For this review, take the finished solid that the model builds, in its own axes (mm). A direction names the side the tool comes from. Coordinates: 2 decimals unless noted, no trailing zeros. Write each loop counter-clockwise with the first axis right and the second up, starting at its lowest first coordinate (ties: lowest second). Pieces come first, ordered by that corner, then holes. Notation, with made-up numbers: (43, -28) -> (82, -28) arc R5 cw to (82, -24) -> close; hole circle Ø4 at (40.25, 27). An arc over 180 degrees is marked (long way). One line per item, written item: value. Start each with the question number.
1) For probe 1 along Y at (x, z) = (-44.5, 2.75); probe 2 along Y at (x, z) = (-35.5, 1); probe 3 along X at (y, z) = (11.5, 0.6), list the stretches that pass through material, from the lowest coordinate up. Write a range as from..to.
2) Add section C-C (z = 1.5). State how many separate pieces and enclosed holes the cut face has, and give its area (3 significant figures).
3) Add section D-D (x = -3.5). State the section outline as (y, z) points, and give its area (3 significant figures).
4) Add section B-B (y = -4.25). State the section outline as (x, z) points, and give its area (3 significant figures).
5) Add section A-A (x = -19.5). State the section outline as (y, z) points.
6) Mouldability with a two-part tool opening along X and no side actions: class faces 1 (the cylindrical face through (-48.87, 23.786, 1.479)), 2 (the cylindrical face through (-33.688, 12.321, 1.479)), 3 (the flat face through (2, 8, 1)), 4 (the flat face through (-44.92, 14.66, 1.48)) as released by +X, released by -X, zero draft, split by the parting line, or undercut.
7) For pin 1 Ø0.9 at (y, z) = (-3.5, 1) entering from -X; pin 2 Ø1 at (y, z) = (0, 2) entering from +X; pin 3 Ø1.5 at (x, z) = (-44.5, 2) entering from +Y, all flat-tipped, find the tip position at first contact; note any pin that passes through.
8) Machinability: for faces 5 (the flat face through (-17, 16.5, 1)), 6 (the flat face through (-41, -2, 1)), 7 (the cylindrical face through (1.4, -24.43, 1.52)), which of the approach directions +Z, -Z, +X, -X, +Y, -Y give a long, thin tool a straight path to every point of the face, cutting with its end or side? Answer none if there is none.
from build123d import *

# Parameters (mm, degrees)
F0_R     = 2
F0_R_2   = 1.9
F0_R_3   = 18.5
F1_DEPTH = 3
F2_R     = 2
F3_R     = 4


with BuildPart() as f1:
    # F0 (on Top) → F1 (new body)
    with BuildSketch(Plane.XY):
        with BuildLine():
            Line((2.0000000052, 16.5001536438), (-35.3637253092, 16.5001536438))
            Line((-35.3637253092, 16.5001536438), (-42.7812429201, 23.375301328))
            ThreePointArc((-42.7812429201, 23.375301328), (-48.9377019653, 23.7146468067), (-48.1133599984, 17.6041964427))
            Line((-48.1133599984, 17.6041964427), (-40.9999999948, 11.0457026558))
            Line((-40.9999999948, 11.0457026558), (-40.9999999948, -17.0001679047))
            Line((-40.9999999948, -17.0001679047), (-45.9997427603, -17.0001679047))
            ThreePointArc((-45.9997427603, -17.0001679047), (-49.9991778461, -21.0673913699), (-45.8653148176, -24.9979084075))
            Line((-45.8653148176, -24.9979084075), (2.0000000052, -24.9998463562))
            Line((2.0000000052, -24.9998463562), (2.0000000052, -16.9998463562))
            Line((2.0000000052, -16.9998463562), (14.0000000052, -16.9998463562))
            Line((14.0000000052, -16.9998463562), (36.0000000052, -16.9998463562))
            Line((36.0000000052, -16.9998463562), (43.2410032397, -23.8966064518))
            ThreePointArc((43.2410032397, -23.8966064518), (48.9041379149, -23.7505294783), (48.7417034391, -18.0878403757))
            Line((48.7417034391, -18.0878403757), (39.0890352428, -8.999838983))
            Line((39.0890352428, -8.999838983), (14.0000000052, -8.999838983))
            Line((14.0000000052, -8.999838983), (2.0000000052, -0.2498463562))
            Line((2.0000000052, -0.2498463562), (2.0000000052, 16.5001536438))
        make_face()
        with Locations((-45.9997427603, -21.0001679047)):
            Circle(F0_R, mode=Mode.SUBTRACT)
        with Locations((-35.5, -20.25)):
            Circle(F0_R_2, mode=Mode.SUBTRACT)
        with Locations((-3.5, -20.25)):
            Circle(F0_R_2, mode=Mode.SUBTRACT)
        with Locations((-19.5, -4.25)):
            Circle(F0_R_3, mode=Mode.SUBTRACT)
        with Locations((45.9997427603, -21.0001679047)):
            Circle(F0_R, mode=Mode.SUBTRACT)
        with Locations((-35.5, 11.75)):
            Circle(F0_R_2, mode=Mode.SUBTRACT)
        with Locations((-3.5, 11.75)):
            Circle(F0_R_2, mode=Mode.SUBTRACT)
        with Locations((-45.9997427603, 21.0001679047)):
            Circle(F0_R, mode=Mode.SUBTRACT)
    extrude(amount=F1_DEPTH)

    # F2
    f2_edges = [f1.edges().sort_by_distance(p)[0] for p in [
        (-41, -17.000168, 1.5),
        (-41, 11.045703, 1.5),
        (-35.363725, 16.500154, 1.5),
        (2, 16.500154, 1.5),
        (2, -16.999846, 1.5),
        (2, -0.249846, 1.5),
        (36, -16.999846, 1.5),
        (2, -24.999846, 1.5),
        (14, -8.999839, 1.5),
    ]]
    fillet(f2_edges, radius=F2_R)

    # F3
    f3_edges = [f1.edges().sort_by_distance(p)[0] for p in [
        (39.089035, -8.999839, 1.5),
    ]]
    fillet(f3_edges, radius=F3_R)


solid = f1.part
Numbers:
1. probe 1: -25..-22.32, -19.68..-17, 14.27..19.68, 22.32..24.71
1. probe 2: -25..-22.15, -18.35..-13.54, 5.04..9.85, 13.65..16.72
1. probe 3: -41.51..-37.38, -33.62..-29.21, -9.79..-5.38, -1.62..2
2. separate pieces: 1
2. enclosed holes: 8
2. area: 1,240 mm²
3. outline: (-25, 0) -> (-22.15, 0) -> (-22.15, 3) -> (-25, 3) -> close; (-18.35, 0) -> (-13.54, 0) -> (-13.54, 3) -> (-18.35, 3) -> close; (5.04, 0) -> (9.85, 0) -> (9.85, 3) -> (5.04, 3) -> close; (13.65, 0) -> (16.5, 0) -> (16.5, 3) -> (13.65, 3) -> close
3. area: 46.0 mm²
4. outline: (-41, 0) -> (-38, 0) -> (-38, 3) -> (-41, 3) -> close; (-1, 0) -> (7.49, 0) -> (7.49, 3) -> (-1, 3) -> close
4. area: 34.5 mm²
5. outline: (-25, 0) -> (-22.75, 0) -> (-22.75, 3) -> (-25, 3) -> close; (14.25, 0) -> (16.5, 0) -> (16.5, 3) -> (14.25, 3) -> close
6. face 1: split by the parting line
6. face 2: undercut
6. face 3: released by +X
6. face 4: released by -X
7. pin 1: x = -41
7. pin 2: x = 2.45
7. pin 3: y = 24.93
8. face 5: +Z, -Z, +X, +Y
8. face 6: +Z, -Z, -X
8. face 7: +Z, -Z, -Y
